The listing builds one solid part. Answer for the finished solid, in the listing's coordinates (mm). A direction names the side the tool comes from. Coordinates: 2 decimals unless noted, no trailing zeros. Loops run counter-clockwise (first coordinate to the right, second up) from the corner with the lowest first, then second, coordinate; pieces in that order, holes last. Notation, with made-up numbers: M 57.5,-25.75 L 94.5,-25.75 A28 ccw 94.5,-2.75 Z; hole C 0,57.25 d5. An arc over 180 degrees is marked long. Return JSON: item names as keys, results as strings. Group by question number.
1. Section D-D (y = 0) is taken. Write down the section's boundary in (x, z).
2. Section A-A (x = 15) is taken. Write down the section's boundary in (y, z), then the cut area to 3 significant figures.
3. Section C-C (z = 2.75) is taken. Write down the section's boundary in (x, y), then the cut area to 3 significant figures.
4. Straight lines are drawn through the part: L1, parallel to Y at x = 2.25, z = 0; L2, parallel to X at y = 10, z = 0; L3, parallel to Y at x = 12.5, z = -1.5. For each, find the intervals that lie inside material, in ascending order. Write a range as from..to.
5. Which of the six approach directions +Z, -Z, +X, -X, +Y, -Y give full straight-line access (tool end or side, diameter ignored) to faces 4 (the face through (-8, 14, 0)), 5 (the face through (-15, 13, 0)), 6 (the face through (3.1, 19.68, 9.14)), 7 (the face through (12, 12, 0)), 8 (the face through (3.1, 19.32, -9.14))?
6. Section B-B (x = -18) is taken. Write down the section's boundary in (y, z), then the cut area to 3 significant figures.
7. Given P1, Ø2.5, axis at x = -15, z = 0, coming from the +Y side; P2, Ø11, axis at x = 16, z = 0.5, coming from the +Y side; P3, Ø7, axis at y = 26, z = -2, coming from the +X side, each flat-ended and moving along its own axis, determine where each tip first touches the part or whether it passes through.
8. The mould has two halves that part along Z. Classify faces 1 (the face through (-14.55, -10.21, -1.43)), 2 (the face through (-14, 32, 7)), 3 (the face through (-5, 8, -10)): pulls with the +Z half, pulls with the -Z half, needs draft (parallel to the pull), parting line crosses it, or undercut.
```python
from build123d import *

# Parameters (mm, degrees)
CROQUIS1_W              = 40
CROQUIS1_H              = 24
CROQUIS1_W_2            = 24
CROQUIS1_H_2            = 20
SALIENTE_EXTRUIR1_DEPTH = 10
CROQUIS3_R              = 8.5
CORTAR_EXTRUIR1_DEPTH   = 70
CROQUIS4_R              = 8.5
CORTAR_EXTRUIR2_DEPTH   = 18
CROQUIS5_R              = 1.5
CORTAR_EXTRUIR3_DEPTH   = 25
CROQUIS6_R              = 1.5
CORTAR_EXTRUIR4_DEPTH   = 30
REDONDEO1_R             = 5
REDONDEO2_R             = 3


with BuildPart() as part:
    # Croquis1 → Saliente-Extruir1 (new, symmetric)
    with BuildSketch(Plane.XY):
        Rectangle(CROQUIS1_W, CROQUIS1_H)
        with Locations((-8, 22)):
            Rectangle(CROQUIS1_W_2, CROQUIS1_H_2)
    extrude(amount=SALIENTE_EXTRUIR1_DEPTH, both=True)

    # Croquis3 → Cortar-Extruir1 (cut)
    with BuildSketch(Plane(origin=(20, 0, 0), x_dir=(0, 0, -1), z_dir=(1, 0, 0))):
        Circle(CROQUIS3_R)
    extrude(amount=-CORTAR_EXTRUIR1_DEPTH, mode=Mode.SUBTRACT)

    # Croquis4 → Cortar-Extruir2 (cut)
    with BuildSketch(Plane(origin=(0, 32, 0), x_dir=(1, 0, 0), z_dir=(0, 1, 0))):
        with Locations(Location((-8, 0, 0), (0, 0, 270))):
            Circle(CROQUIS4_R)
    extrude(amount=-CORTAR_EXTRUIR2_DEPTH, mode=Mode.SUBTRACT)

    # Croquis5 → Cortar-Extruir3 (cut)
    with BuildSketch(Plane.XZ.offset(12)):
        with Locations(Location((-15, 0, 0), (0, 0, 270))):
            Circle(CROQUIS5_R)
        with Locations(Location((15, 0, 0), (0, 0, 270))):
            Circle(CROQUIS5_R)
    extrude(amount=-CORTAR_EXTRUIR3_DEPTH, mode=Mode.SUBTRACT)

    # Croquis6 → Cortar-Extruir4 (cut)
    with BuildSketch(Plane.ZY.offset(20)):
        with Locations(Location((0, 24, 0), (0, 0, 270))):
            Circle(CROQUIS6_R)
    extrude(amount=-CORTAR_EXTRUIR4_DEPTH, mode=Mode.SUBTRACT)

    # Redondeo1
    redondeo1_edges = [part.edges().sort_by_distance(p)[0] for p in [
        (0, -12, -10),
        (12, 12, 10),
        (0, -12, 10),
        (12, 12, -10),
    ]]
    fillet(redondeo1_edges, radius=REDONDEO1_R)

    # Redondeo2
    redondeo2_edges = [part.edges().sort_by_distance(p)[0] for p in [
        (4, 19.5, 10),
        (4, 19.5, -10),
    ]]
    fillet(redondeo2_edges, radius=REDONDEO2_R)


solid = part.part
```
Worked out:
{
 "1": {"outline": "M -20,-10 L 20,-10 L 20,-8.5 L -20,-8.5 Z; M -20,8.5 L 20,8.5 L 20,10 L -20,10 Z"},
 "2": {"outline": "M -12,-5 A5 ccw -7,-10 L 7,-10 A5 ccw 12,-5 L 12,-1.5 L 8.37,-1.5 A8.5 cw -8.37,-1.5 L -12,-1.5 Z; M -12,1.5 L -8.37,1.5 A8.5 cw 8.37,1.5 L 12,1.5 L 12,5 A5 ccw 7,10 L -7,10 A5 ccw -12,5 Z", "area": "210 mm^2"},
 "3": {"outline": "M -20,-12 L 20,-12 L 20,-8.04 L -20,-8.04 Z; M -20,8.04 L 20,8.04 L 20,12 L 4,12 L 4,32 L 0.04,32 L 0.04,14 L -16.04,14 L -16.04,32 L -20,32 Z", "area": "507 mm^2"},
 "4": {"L1": "-12..-8.5, 8.5..22.5, 25.5..32", "L2": "-20..-16.5, -13.5..13.5, 16.5..20", "L3": "-12..-8.37, 8.37..12"},
 "5": {"face 4": "+Y", "face 5": "-Y", "face 6": "+Z, +X, +Y", "face 7": "+Z, -Z, +X, +Y", "face 8": "-Z, +X, +Y"},
 "6": {"outline": "M -12,-5 A5 ccw -7,-10 L 32,-10 L 32,10 L -7,10 A5 ccw -12,5 Z; hole C 0,0 d17; hole C 24,0 d3", "area": "635 mm^2"},
 "7": {"P1": "y = 14", "P2": "y = 12", "P3": "x = 4"},
 "8": {"face 1": "undercut", "face 2": "needs draft", "face 3": "pulls with the -Z half"}
}
